Work out the finished part from the listing and answer in its coordinate system (mm). A direction names the side the tool comes from. Round coordinates to 2 decimals unless told otherwise and drop trailing zeros. Order: outer loops, then holes, each group sorted by start corner. A loop starts at its lowest first (then second) coordinate and runs counter-clockwise, first axis right, second up. Notation, with made-up numbers: M 49.5,19 L 107.5,19 A27 cw 107.5,44 Z; hole C 18,51.5 d7. An arc over 180 degrees is marked long. Return JSON: item names as keys, results as strings.
Autodesk Inventor part; units mm, degrees
ref_plane "YZ Plane" through (0, 0, 0) normal (1, 0, 0) x (0, 1, 0)
ref_plane "XZ Plane" through (0, 0, 0) normal (0, 1, 0) x (-1, 0, 0)
ref_plane "XY Plane" through (0, 0, 0) normal (0, 0, 1) x (1, 0, 0)
sketch "Sketch1" plane through (0, 0, 0) normal (0, 1, 0) x (-1, 0, 0)
  line L0 (0, 0) -> (10, 0)
  line L1 (10, 0) -> (10, -10)
  line L2 (10, -10) -> (0, -10)
  line L3 (0, -10) -> (0, 0)
  dimension "d0" = 10
  dimension "d1" = 10
extrude "Extrusion1" add sketch "Sketch1" along normal blind 3.36
sketch "Sketch2" plane through (0, 3.36, 0) normal (0, 1, 0) x (1, 0, 0)
  line L0 (-10, 10) -> (-10, 0)
  circle A0 centre (-5, 5) radius 1.37
  point P0 (0, 0)
  dimension "d4" = 2.74
extrude "Extrusion2" cut sketch "Sketch2" against normal blind 3.36
sketch "Sketch3" plane through (0, 3.36, 0) normal (0, 1, 0) x (1, 0, 0)
  line L0 (-10, 10) -> (-10, 0)
  circle A0 centre (-5, 5) radius 2.75
  circle A1 centre (-5, 5) radius 4.475
  point P0 (0, 0)
  dimension "d7" = 5.5
  dimension "d8" = 8.95
extrude "Extrusion3" add sketch "Sketch3" along normal blind 3
sketch "Sketch4" plane through (0, 0, 0) normal (0, -1, 0) x (1, 0, 0)
  line L0 (-1.2, 0) -> (-1.2, -10)
  line L1 (-8.8, 0) -> (-8.8, -10)
  line L2 (-1.2, -10) -> (-8.8, -10)
  line L3 (0, -10) -> (-10, -10)
  line L4 (-8.8, 0) -> (-1.2, 0)
  line L5 (-10, 0) -> (0, 0)
  dimension "d11" = 1.2
extrude "Extrusion4" cut sketch "Sketch4" against normal blind 2.16
properties part number "MMAE 232 Assignment 2_Servo Horn 2 - Dylan Tamras"
Item 1: Find section C-C (x = -5). Determine the outline of the cut face in (y, z) (3 decimals).
Output:
{"outline": "M 2.16,-10 L 3.36,-10 L 3.36,-9.475 L 6.36,-9.475 L 6.36,-7.75 L 3.36,-7.75 L 3.36,-6.37 L 2.16,-6.37 Z; M 2.16,-3.63 L 3.36,-3.63 L 3.36,-2.25 L 6.36,-2.25 L 6.36,-0.525 L 3.36,-0.525 L 3.36,0 L 2.16,0 Z"}
Item 2: Find section D-D (y = 3). Determine the outline of the cut face in (x, z).
Output:
{"outline": "M -10,-10 L 0,-10 L 0,0 L -10,0 Z; hole C -5,-5 d2.74"}
Item 3: This flat-tipped pin is pushed along its axis until it touches: pin 1 (2.5 mm diameter, centred on y = 1, z = -5, fed in from +X). Where does it stop, or does it pass through?
Output:
{"pin 1": "stops at x = 0"}
Item 4: Consider line 1 along X through (y, z) = (5, -5) (3 decimals); line 2 along X through (y, z) = (1.5, -9); line 3 along Z through (x, y) = (-5, 2.85). Determine where each line is inside the solid, lowest interval first. Write a range as [from, to].
Output:
{"line 1": "x = [-9.475, -7.75], [-2.25, -0.525]", "line 2": "x = [-10, -8.8], [-1.2, 0]", "line 3": "z = [-10, -6.37], [-3.63, 0]"}
Item 5: Find section B-B (y = 2). Determine the outline of the cut face in (x, z).
Output:
{"outline": "M -10,-10 L -8.8,-10 L -8.8,0 L -10,0 Z; M -1.2,-10 L 0,-10 L 0,0 L -1.2,0 Z"}
Item 6: Which of the six approach directions +Z, -Z, +X, -X, +Y, -Y give full straight-line access (tool end or side, diameter ignored) to faces 4 (the flat face through (-1.2, 1, -5)), 5 (the flat face through (0, 2, -5)), 6 (the cylindrical face through (-3.73, 4.84, -7.44))?
Output:
{"face 4": "+Z, -Z, -Y", "face 5": "+Z, -Z, +X, +Y, -Y", "face 6": "+Y"}
Item 7: The mould has two halves that part along Z. Classify faces 1 (the flat face through (-7, 2.16, -5)), 2 (the flat face through (-6.2, 3.36, -6.2)), 3 (the flat face through (-5.1, 2.4, -10)): pulls with the +Z half, pulls with the -Z half, needs draft (parallel to the pull), parting line crosses it, or undercut.
Output:
{"face 1": "needs draft", "face 2": "undercut", "face 3": "pulls with the -Z half"}
Item 8: Find section A-A (z = -5). Determine the outline of the cut face in (x, y) (3 decimals).
Output:
{"outline": "M -10,0 L -8.8,0 L -8.8,2.16 L -6.37,2.16 L -6.37,3.36 L -7.75,3.36 L -7.75,6.36 L -9.475,6.36 L -9.475,3.36 L -10,3.36 Z; M -3.63,2.16 L -1.2,2.16 L -1.2,0 L 0,0 L 0,3.36 L -0.525,3.36 L -0.525,6.36 L -2.25,6.36 L -2.25,3.36 L -3.63,3.36 Z"}
